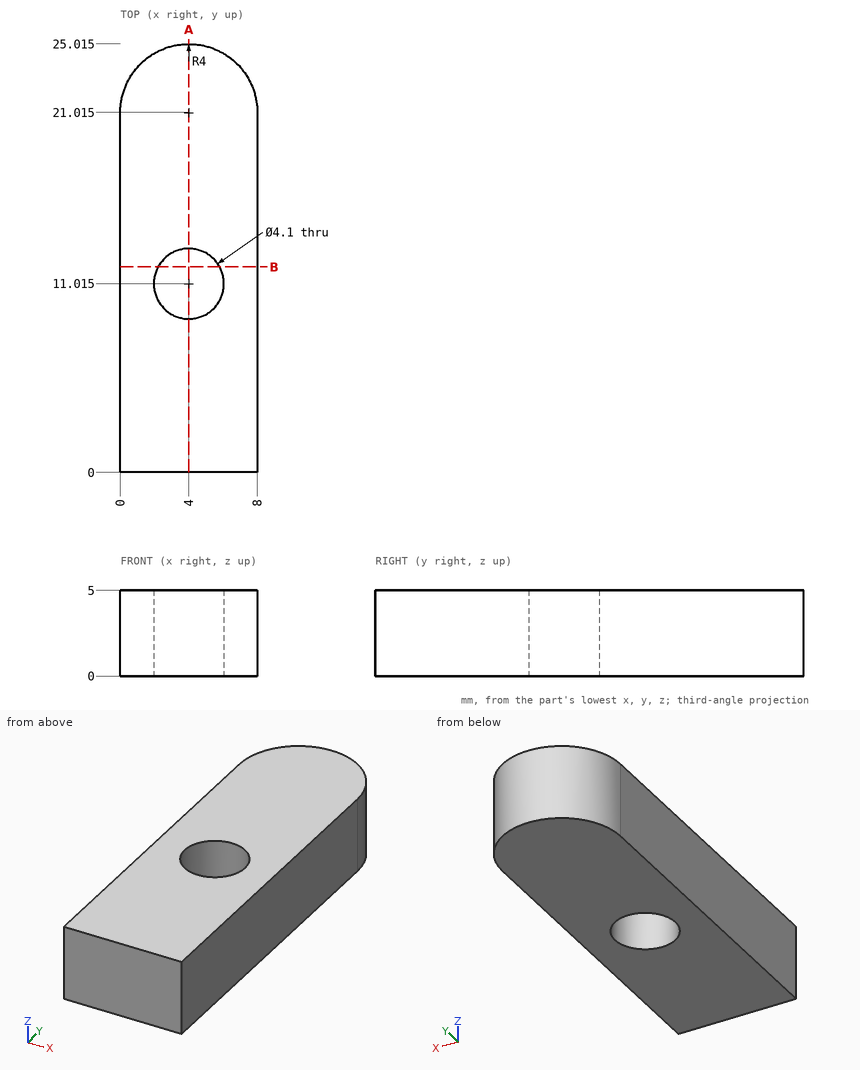
Can you work these out from the drawing? Everything is in mm from the part's minimum corner. Give positions to 0.01 mm unless a question says otherwise; leave off trailing zeros. Order: outer loops, then holes, each group sorted by start corner. A loop starts at its lowest first (then second) coordinate and runs counter-clockwise, first axis right, second up. Notation, with made-up numbers: M 45,83.5 L 72,83.5 A23 ccw 72,95.5 Z; hole C 79.25,85 d5. An arc over 180 degrees is marked long. One line per question, with ' | ' between items.
1. I want a section at A-A (x = 4). List the corners of the cut face in (y, z) for me (1 decimal).
Results:
outline: M 0,0 L 9,0 L 9,5 L 0,5 Z; M 13.1,0 L 25,0 L 25,5 L 13.1,5 Z
2. If I drill on line 1 (Y direction, x = 4, z = 3.5) (1 decimal); line 2 (Y direction, x = 3.75, z = 4.3); line 3 (X direction, y = 10.75, z = 1.8), over which ranges is the centre line in solid material (lowest first)?
Results:
line 1: 0 to 9, 13.1 to 25 | line 2: 0 to 8.98, 13.05 to 25.01 | line 3: 0 to 1.97, 6.03 to 8
3. I want a section at B-B (y = 12). List the corners of the cut face in (x, z) for me.
Results:
outline: M 0,0 L 2.2,0 L 2.2,5 L 0,5 Z; M 5.8,0 L 8,0 L 8,5 L 5.8,5 Z
